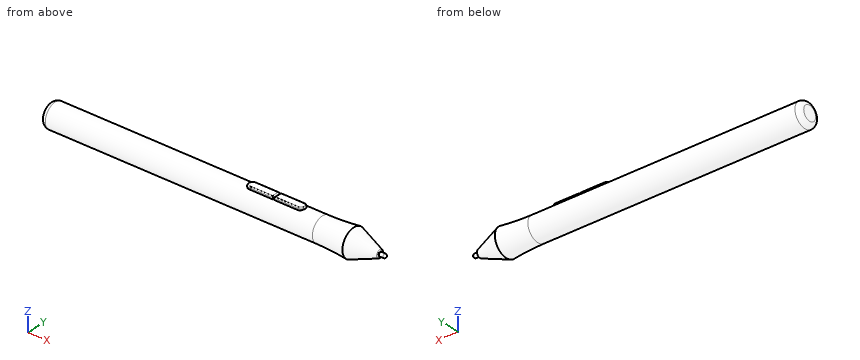
Autodesk Fusion 360 part; units mm, degrees
sketch "Sketch1" plane through (0, 0, 0) normal (0, 1, 0) x (1, 0, 0)
  line L0 (-138.8, 0) -> (-138.8, 3)
  arc A0 (-136.8, 5) -> (-138.8, 3) centre (-136.8, 3) ccw
  line L1 (-136.8, 5) -> (-26.5, 5)
  arc A1 (-26.5, 5) -> (-13.5, 5.75) centre (-26.5, 118.0417) ccw
  line L2 (-13.5, 5.75) -> (-2.5, 1.5)
  line L3 (-2.5, 1.5) -> (-2.5, 0.8)
  line L4 (-2.5, 0.8) -> (-0.8, 0.8)
  arc A2 (0, 0) -> (-0.8, 0.8) centre (-0.8, 0) ccw
  line L5 (0, 5) -> (0, -5) construction
  line L6 (1.75, 0) -> (22.5, 0)
  line L7 (-138.8, 0) -> (0, 0)
  dimension "d1" = 0.8
  dimension "d2" = 2.5
  dimension "d3" = 1.5
  dimension "d4" = 11
  dimension "d5" = 5.75
  dimension "d6" = 5
  dimension "d7" = 13
  dimension "d8" = 3
  dimension "d9" = 125.3
revolve "Revolve1" add sketch "Sketch1" angle 360 about axis through (1.75, 0, 0) along (1, 0, 0)
sketch "Sketch2" plane through (0, 0, 0) normal (0, 0, 1) x (1, 0, 0)
  line L0 (-45, 1.75) -> (-45, -1.75)
  line L1 (-45, -1.75) -> (-35.25, -1.75)
  arc A0 (-35.25, -1.75) -> (-35.25, 1.75) centre (-35.25, 0) ccw
  line L2 (-35.25, 1.75) -> (-45, 1.75)
  line L3 (-45.5, 1.75) -> (-45.5, -1.75)
  line L4 (-45.5, -1.75) -> (-55.25, -1.75)
  arc A1 (-55.25, 1.75) -> (-55.25, -1.75) centre (-55.25, 0) ccw
  line L5 (-55.25, 1.75) -> (-45.5, 1.75)
  line L6 (-57, 0) -> (-33.5, 0) construction
  point P0 (-13.5, 0)
  dimension "d11" = 0.5
  dimension "d12" = 3.5
  dimension "d13" = 23.5
  dimension "d14" = 20
extrude "Extrude1" add sketch "Sketch2" along normal blind 5.75
fillet "Fillet1" radius 0.4 8 edges at (-40.125, -1.75, 5.75) (-33.5, 0, 5.75) (-40.125, 1.75, 5.75) (-50.375, 1.75, 5.75) (-57, 0, 5.75) (-50.375, -1.75, 5.75) (-45.5, 0, 5.75) (-45, 0, 5.75)
fillet "Fillet1" radius 0.4 1 edges at (-2.5, -0.5424, 1.3985)
Build history of the part. All positions in model axes, mm. Coordinates: 2 decimals unless noted, no trailing zeros. Order: outer loops, then holes, each group sorted by start corner. A loop starts at its lowest first (then second) coordinate and runs counter-clockwise, first axis right, second up. Notation, with made-up numbers: (-2.5, -23) -> (7.5, -23) arc R25 ccw to (7.5, 16) -> close; hole circle Ø5 at (13, -12). An arc over 180 degrees is marked (long way). Answer in a Markdown table with one row per item. Add a question column.
Q1. Band-saw the part on A-A, the plane x = -40. List the corners of the cut face in (y, z), then the cut area to 3 significant figures.
Q2. Drop flat-ended pins along their axis: pin 1 (0.5 mm diameter, centred on x = -52, z = 5, fed in from +Y); pin 2 (2 mm diameter, centred on x = -50.5, y = 3, fed in from -Z); pin 3 (1 mm diameter, centred on x = -73, y = 4, fed in from -Z). Give the stop position or say it passes through.
Q3. Wall check: line 1 along Y through (x, z) = (-68, 4); line 2 along X through (y, z) = (-0.5, -1); line 3 along Y through (x, z) = (-54.5, 0.5). Give the ranges that are in metal, low to high. Write a range as [from, to].
Q4. Band-saw the part on B-B, the plane x = -21. List the corners of the cut face in (y, z).
Answers follow:
| question | item | result |
|---|---|---|
| 1 | outline | (-1.75, 4.68) arc R5 ccw (long way) to (1.75, 4.68) -> (1.75, 5.35) arc R0.4 ccw to (1.35, 5.75) -> (-1.35, 5.75) arc R0.4 ccw to (-1.75, 5.35) -> close |
| 1 | area | 81.5 mm^2 |
| 2 | pin 1 | y = 1.75 |
| 2 | pin 2 | z = -4.58 |
| 2 | pin 3 | z = -3.57 |
| 3 | line 1 | [-3, 3] |
| 3 | line 2 | [-138.8, -2.5] |
| 3 | line 3 | [-4.97, 4.97] |
| 4 | outline | circle Ø10.27 at (0, 0) |
